Build history of the part. All positions in model axes, mm. Face numbers are marked on the shaded views. A direction names the side the tool comes from. Round coordinates to 2 decimals unless told otherwise and drop trailing zeros. Write each loop counter-clockwise with the first axis right and the second up, starting at its lowest first coordinate (ties: lowest second). Pieces come first, ordered by that corner, then holes. Notation, with made-up numbers: M -11.5,-20 L 0.5,-20 A34 ccw 0.5,15 Z; hole C 87,-28 d8. An arc over 180 degrees is marked long. Use a Markdown table: item, result.
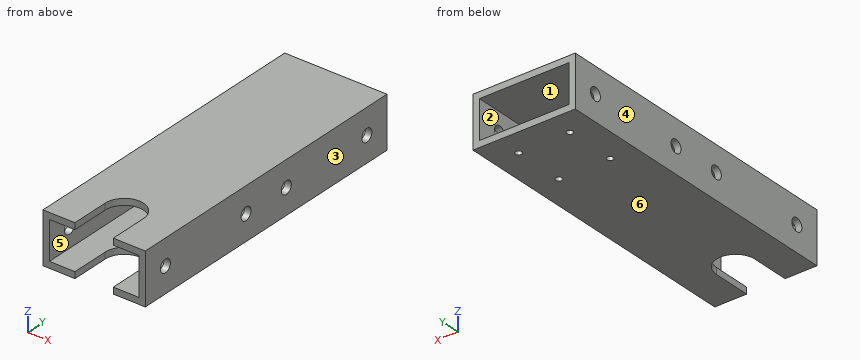
Autodesk Inventor part; units mm, degrees
ref_plane "YZ Plane" through (0, 0, 0) normal (1, 0, 0) x (0, 1, 0)
ref_plane "XZ Plane" through (0, 0, 0) normal (0, 1, 0) x (-1, 0, 0)
ref_plane "XY Plane" through (0, 0, 0) normal (0, 0, 1) x (1, 0, 0)
sketch "Sketch1" plane through (0, 0, 0) normal (0, 1, 0) x (-1, 0, 0)
  line L0 (0, 0) -> (-50.8, 0)
  line L1 (-50.8, 0) -> (-50.8, -25.4)
  line L2 (-50.8, -25.4) -> (0, -25.4)
  line L3 (0, -25.4) -> (0, 0)
  line L4 (-3.175, -22.225) -> (-47.625, -22.225)
  line L5 (-47.625, -22.225) -> (-47.625, -3.175)
  line L6 (-47.625, -3.175) -> (-3.175, -3.175)
  line L7 (-3.175, -3.175) -> (-3.175, -22.225)
  dimension "d0" = 50.8
  dimension "d1" = 25.4
  dimension "d2" = 44.45
  dimension "d3" = 19.05
  dimension "d4" = 3.175
  dimension "d5" = 3.175
extrude "Extrusion1" add sketch "Sketch1" along normal blind 152.4
sketch "Sketch2" plane through (0, 0, -25.4) normal (-1, 0, 0) x (0, 0, 1)
  line L0 (22.225, 152.4) -> (3.175, 152.4)
  line L1 (12.7, 152.4) -> (12.7, 0) construction
  line L2 (3.175, 0) -> (22.225, 0)
  line L3 (0, 0) -> (0, 152.4) construction
  line L4 (25.4, 0) -> (25.4, 152.4) construction
  line L5 (25.4, 0) -> (25.4, 152.4)
  line L6 (25.4, 76.2) -> (0, 76.2) construction
  circle A0 centre (12.7, 88.9) radius 3.175
  circle A1 centre (12.7, 63.5) radius 3.175
  circle A2 centre (12.7, 139.7) radius 3.175
  circle A3 centre (12.7, 12.7) radius 3.175
  dimension "d8" = 6.35
  dimension "d9" = 12.7
  dimension "d10" = 6.35
  dimension "d11" = 12.7
hole "Hole2" at (0, 139.7, -12.7) at (0, 88.9, -12.7) at (0, 63.5, -12.7) at (0, 12.7, -12.7) direction (1, 0, 0) diameter 6.35 end through all
sketch "Sketch3" plane through (50.8, 0, -25.4) normal (0, 0, -1) x (-1, 0, 0)
  line L0 (50.8, 152.4) -> (0, 152.4)
  line L1 (25.4, 152.4) -> (25.4, 0) construction
  line L2 (12.7, 152.4) -> (12.7, 139.7) construction
  line L3 (0, 0) -> (0, 152.4)
  line L4 (0, 127) -> (50.8, 127) construction
  circle A0 centre (12.7, 139.7) radius 1.5875
  circle A1 centre (38.1, 139.7) radius 1.5875
  circle A2 centre (12.7, 114.3) radius 1.5875
  circle A3 centre (38.1, 114.3) radius 1.5875
  point P0 (50.8, 0)
  dimension "d27" = 12.7
  dimension "d28" = 12.7
  dimension "d30" = 3.175
  dimension "d31" = 25.4
hole "Hole3" at (38.1, 139.7, -25.4) at (38.1, 114.3, -25.4) at (12.7, 114.3, -25.4) at (12.7, 139.7, -25.4) direction (0, 0, 1) diameter 3.175 depth 3.175 tip angle 118
sketch "Sketch4" plane through (0, 0, 0) normal (0, 0, 1) x (1, 0, 0)
  line L0 (0, 0) -> (50.8, 0)
  line L1 (34.925, 0) -> (34.925, 19.05)
  line L2 (15.875, 0) -> (15.875, 19.05)
  line L3 (0, 0) -> (0, 152.4)
  line L4 (50.8, 0) -> (50.8, 152.4)
  circle A0 centre (25.4, 19.05) radius 9.525
  line L5 (15.875, 0) -> (34.925, 0)
  line L6 (47.625, 0) -> (3.175, 0)
  line L7 (15.875, 19.05) -> (34.925, 19.05)
  line L8 (34.925, 19.05) -> (34.925, 0)
  line L9 (34.925, 0) -> (15.875, 0)
  line L10 (15.875, 0) -> (15.875, 19.05)
  dimension "d39" = 15.875
  dimension "d40" = 15.875
  dimension "d48" = 19.05
  dimension "d49" = 19.05
hole "Hole4" at (25.4, 19.05, 0) direction (0, 0, -1) diameter 19.05 depth 25.4 tip angle 118
extrude "Extrusion2" cut sketch "Sketch4" against normal blind 25.4 contours L2 A0 L1 L0 | L7 A0 picked at (22.9312, 16.1848)
properties part number "2AM-17-P-0205" material "Aluminum 6061"
Q1. Which spindle directions (+Z, -Z, +X, -X, +Y, -Y) get a long thin tool onto all of the face, cutting with end or side? Do the marked faces 5 and 6. Say none if no direction does.
Response values:
| item | result |
|---|---|
| face 5 | +Y, -Y |
| face 6 | -Z, +X, -X, +Y, -Y |
Q2. Cut at A-A on z = -5.75. Give the cut face in (x, y) (3 decimals), and give its area (3 significant figures).
Response values:
| item | result |
|---|---|
| outline | M 0,0 L 3.175,0 L 3.175,152.4 L 0,152.4 Z; M 47.625,0 L 50.8,0 L 50.8,152.4 L 47.625,152.4 Z |
| area | 968 mm2 |
Q3. Cut at C-C on x = 25.4. Give the cut face in (y, z) (3 decimals), and give its area (3 significant figures).
Response values:
| item | result |
|---|---|
| outline | M 28.575,-25.4 L 152.4,-25.4 L 152.4,-22.225 L 28.575,-22.225 Z; M 28.575,-3.175 L 152.4,-3.175 L 152.4,0 L 28.575,0 Z |
| area | 786 mm2 |
Q4. Drill centre lines: L1, parallel to X at y = 114.3, z = -23.3; L2, parallel to Y at x = 12.7, z = -24.05; L3, parallel to Y at x = 1.6, z = -12.7 (3 decimals). Where is each one in solid material? Low to high.
Response values:
| item | result |
|---|---|
| L1 | x = 0 to 11.11, 14.29 to 36.51, 39.69 to 50.8 |
| L2 | y = 0 to 112.71, 115.89 to 138.11, 141.29 to 152.4 |
| L3 | y = 0 to 9.525, 15.875 to 60.325, 66.675 to 85.725, 92.075 to 136.525, 142.875 to 152.4 |
Q5. Two-plate mould, pull along X, no slides. Class the marked faces 1, 2, 3 and 4: +X half, -X half, draft (parallel to the pull), parting line (faces both ways), or undercut.
Response values:
| item | result |
|---|---|
| face 1 | undercut |
| face 2 | undercut |
| face 3 | +X half |
| face 4 | -X half |
Q6. Drop a flat-ended pin along its axis: P1, Ø5.5, axis at y = 88.9, z = -12.7, coming from the -X side. Give the stop position or say it passes through.
Response values:
| item | result |
|---|---|
| P1 | passes through |
Q7. Cut at B-B on y = 63.5. Give the cut face in (x, z) (3 decimals).
Response values:
| item | result |
|---|---|
| outline | M 0,-25.4 L 50.8,-25.4 L 50.8,-15.875 L 47.625,-15.875 L 47.625,-22.225 L 3.175,-22.225 L 3.175,-15.875 L 0,-15.875 Z; M 0,-9.525 L 3.175,-9.525 L 3.175,-3.175 L 47.625,-3.175 L 47.625,-9.525 L 50.8,-9.525 L 50.8,0 L 0,0 Z |
Q8. Cut at D-D on y = 139.7. Give the cut face in (x, z) (1 decimal).
Response values:
| item | result |
|---|---|
| outline | M 0,-25.4 L 11.1,-25.4 L 11.1,-22.2 L 3.2,-22.2 L 3.2,-15.9 L 0,-15.9 Z; M 0,-9.5 L 3.2,-9.5 L 3.2,-3.2 L 47.6,-3.2 L 47.6,-9.5 L 50.8,-9.5 L 50.8,0 L 0,0 Z; M 14.3,-25.4 L 36.5,-25.4 L 36.5,-22.2 L 14.3,-22.2 Z; M 39.7,-25.4 L 50.8,-25.4 L 50.8,-15.9 L 47.6,-15.9 L 47.6,-22.2 L 39.7,-22.2 Z |
